Geometry check sheet. Reference: drawing and pictorial views, mm from the part's lowest x, y, z. A direction names the side the tool comes from. Coordinates: 2 decimals unless noted, no trailing zeros. Write each loop counter-clockwise with the first axis right and the second up, starting at its lowest first coordinate (ties: lowest second). Pieces come first, ordered by that corner, then holes. Notation, with made-up numbers: (16.25, 39.25) - (60.25, 39.25) arc R25 cw to (60.25, 68.25) - close; hole circle Ø4 at (14.25, 7.25). An arc over 180 degrees is marked (long way). Answer as a JSON object with one key per item and string values. Group by question number.
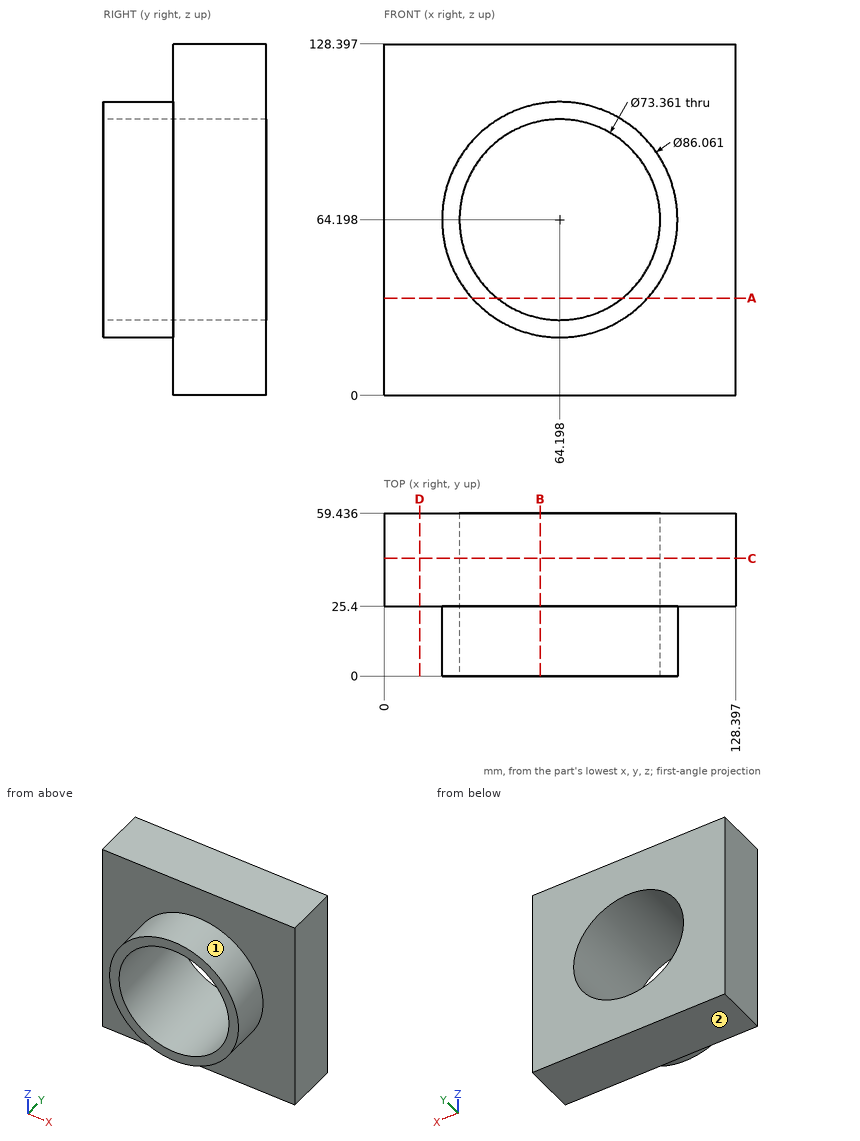
(1) Section check D-D (x = 13). Record the cut outline in (y, z).
(2) Gauge pin test, flat ends, axial feed: pin 1 (12 mm diameter, centred on x = 64.5, z = 20, fed in from -Y); pin 2 (10 mm diameter, centred on y = 19.5, z = 107, fed in from -X); pin 3 (3 mm diameter, centred on y = 18.5, z = 102.5, fed in from -X). Record the tip position at first contact, or that the pin passes through.
(3) Material ranges on L1, parallel to Y at x = 72, z = 116; L2, parallel to X at y = 26, z = 64.5; L3, parallel to Z at x = 62.5, y = 29.5, recorded low to high. Write a range as [from, to].
(4) Section check B-B (x = 57). Record the cut outline in (y, z) (1 decimal), and give its area (3 significant figures).
(5) Set-up check for the marked faces 1 and 2: record each of +Z, -Z, +X, -X, +Y, -Y from which the full face is reachable in a straight line by a thin tool's end or side.
(6) Section check C-C (y = 43). Record the cut outline in (x, z), and give its area (3 significant figures).
(7) Section check A-A (z = 35.5). Record the cut outline in (x, y) (1 decimal).
Conclusion:
{
 "1": {"outline": "(25.4, 0) - (59.44, 0) - (59.44, 128.4) - (25.4, 128.4) - close"},
 "2": {"pin 1": "stops at y = 0", "pin 2": "stops at x = 43.64", "pin 3": "stops at x = 41.9"},
 "3": {"L1": "y = [25.4, 59.44]", "L2": "x = [0, 27.52], [100.88, 128.4]", "L3": "z = [0, 27.56], [100.84, 128.4]"},
 "4": {"outline": "(0, 21.8) - (25.4, 21.8) - (25.4, 0) - (59.4, 0) - (59.4, 28.2) - (0, 28.2) - close; (0, 100.2) - (59.4, 100.2) - (59.4, 128.4) - (25.4, 128.4) - (25.4, 106.6) - (0, 106.6) - close", "area": "2,250 mm^2"},
 "5": {"face 1": "-Y", "face 2": "-Z, +X, -X, +Y, -Y"},
 "6": {"outline": "(0, 0) - (128.4, 0) - (128.4, 128.4) - (0, 128.4) - close; hole circle Ø73.36 at (64.2, 64.2)", "area": "12,300 mm^2"},
 "7": {"outline": "(0, 25.4) - (32.1, 25.4) - (32.1, 0) - (41.4, 0) - (41.4, 59.4) - (0, 59.4) - close; (87, 0) - (96.3, 0) - (96.3, 25.4) - (128.4, 25.4) - (128.4, 59.4) - (87, 59.4) - close"}
}
